Input: part model. Units: mm. Frame: model coordinates. A direction names the side the tool comes from. Coordinates: 2 decimals unless noted, no trailing zeros. Write each loop counter-clockwise with the first axis right and the second up, starting at its lowest first coordinate (ties: lowest second). Pieces come first, ordered by that corner, then holes. Notation, with made-up numbers: (59.5, 54) -> (83.5, 54) arc R17 ccw to (83.5, 80) -> close; hole circle Ø6 at (49.5, 33). An arc over 180 degrees is marked (long way). One line per question, with ' | ' between items. Start each with the question number.
Autodesk Inventor part; units mm, degrees
ref_plane "Arbeitsebene1" through (35.8206, 9.157, 7) normal (0, 0, -1) x (0, 1, 0)
ref_plane "Arbeitsebene2" through (35.8206, 9.157, -7) normal (0, 0, 1) x (1, 0, 0)
ref_plane "YZ Plane" through (0, 0, 0) normal (1, 0, 0) x (0, 1, 0)
sketch "Skizze1" plane through (0, 0, 0) normal (0, 0, 1) x (1, 0, 0)
  circle A0 centre (13.3363, -13.3273) radius 2.25
  circle A1 centre (69.9048, -13.3273) radius 2.25
  line L0 (49.1839, 14.957) -> (45.4022, 8.407)
  line L1 (45.4022, 8.407) -> (37.8389, 8.407)
  line L2 (37.8389, 8.407) -> (34.0573, 14.957)
  circle A2 centre (-86.3794, -2.543) radius 2.1
  line L3 (-65.3794, -2.3212) -> (-80.3794, -2.3212)
  line L4 (-80.3794, -2.3212) -> (-80.3794, 8.457)
  line L5 (-80.3794, 8.457) -> (-86.3794, 8.457)
  line L6 (-86.3794, 8.457) -> (-86.3794, 3.857)
  line L7 (-86.3794, 3.857) -> (-93.3794, 3.857)
  line L8 (-93.3794, 3.857) -> (-93.3794, 8.457)
  line L9 (-93.3794, 8.457) -> (-98.3794, 8.457)
  line L10 (-98.3794, 8.457) -> (-98.3794, -15.043)
  line L11 (-38.3794, -15.043) -> (-98.3794, -15.043)
  spline S0 degree 3 poles (16.2456, -28.9938) (-0.41, -19.3777) (-19.1473, -15.043) (-38.3794, -15.043) knots 1 1 1 1 2 2 2 2
  arc A3 (16.2456, -28.9938) -> (92.3706, 14.957) centre (41.6206, 14.957) ccw
  line L12 (-93.3794, 21.457) -> (-98.3794, 21.457)
  line L13 (-93.3794, 21.457) -> (-93.3794, 26.057)
  line L14 (-93.3794, 26.057) -> (-86.3794, 26.057)
  line L15 (-86.3794, 26.057) -> (-86.3794, 21.457)
  line L16 (-86.3794, 21.457) -> (-80.3794, 21.457)
  line L17 (-80.3794, 32.2352) -> (-80.3794, 21.457)
  line L18 (-65.3794, -4.043) -> (-65.3794, -2.3212)
  line L19 (26.6206, 28.1857) -> (26.6206, 1.7282)
  line L20 (26.6206, 1.7282) -> (16.7234, -4.043)
  line L21 (16.7234, -4.043) -> (-65.3794, -4.043)
  circle A4 centre (41.6206, 14.957) radius 4.1 construction
  line L22 (46.3548, 14.957) -> (43.9877, 19.057)
  line L23 (43.9877, 19.057) -> (39.2534, 19.057)
  line L24 (39.2534, 19.057) -> (36.8863, 14.957)
  line L25 (36.8863, 14.957) -> (39.2534, 10.857)
  line L26 (39.2534, 10.857) -> (43.9877, 10.857)
  line L27 (43.9877, 10.857) -> (46.3548, 14.957)
  arc A5 (92.3706, 14.957) -> (16.2456, 58.9078) centre (41.6206, 14.957) ccw
  spline S1 degree 3 poles (16.2456, 58.9078) (-0.41, 49.2917) (-19.1473, 44.957) (-38.3794, 44.957) knots 1 1 1 1 2 2 2 2
  line L28 (-38.3794, 44.957) -> (-98.3794, 44.957)
  line L29 (-98.3794, 21.457) -> (-98.3794, 44.957)
  line L30 (-65.3794, 32.2352) -> (-80.3794, 32.2352)
  line L31 (-65.3794, 33.957) -> (-65.3794, 32.2352)
  line L32 (16.7234, 33.957) -> (-65.3794, 33.957)
  line L33 (26.6206, 28.1857) -> (16.7234, 33.957)
  circle A6 centre (13.3363, 43.2412) radius 2.25
  circle A7 centre (69.9048, 43.2412) radius 2.25
  circle A8 centre (-86.3794, 32.457) radius 2.1
  line L34 (37.8389, 21.507) -> (34.0573, 14.957)
  line L35 (45.4022, 21.507) -> (37.8389, 21.507)
  line L36 (49.1839, 14.957) -> (45.4022, 21.507)
  point P0 (0, 0)
  dimension "d0" = 8.2
ref_plane "Arbeitsebene1" through (35.8206, 9.157, 7) normal (0, 0, -1) x (0, 1, 0)
ref_plane "Arbeitsebene2" through (35.8206, 9.157, -7) normal (0, 0, 1) x (1, 0, 0)
extrude "Extrusion1" add sketch "Skizze1" against normal up to surface (14 mm away) from surface at 7 contours L0 L1 L2 L34 L35 L36
properties part number "Nutspacker" material "ABS-Kunststoff - Schwarz"
1) First-contact query: P1, Ø3, axis at x = 41, y = 16, coming from the +Z side; P2, Ø2, axis at y = 19.5, z = -4, coming from the -X side. Flat tips, straight axial feed; report the tip coordinate or a pass-through.
2) Access query for faces 1 (the face through (42, 8.407, 0)), 2 (the face through (38.05, 12.94, 0.1)). Directions: +Z, -Z, +X, -X, +Y, -Y. A direction counts if a zero-diameter tool reaches every point of the face in a straight line with its end or side. Return the directions, or none.
3) Section D-D, the plane x = 36. Return loops of the section in (y, z).
4) Section A-A, the plane z = 4.75. Return loops of the section in (x, y).
5) Pull-direction query (X, two-part tool) for faces 3 (the face through (42, 10.857, 0)), 4 (the face through (42, 21.507, 0)), 5 (the face through (47.32, 11.73, 0.1)); classes: released by +X, released by -X, zero draft, split by the parting line, or undercut.
6) Section B-B, the plane x = 42. Return loops of the section in (y, z).
7) Ray query, line 1 (Y direction, x = 40, z = 2.75); line 2 (X direction, y = 12.5, z = -4.5); line 3 (X direction, y = 16.25, z = 3.75). Return the intervals inside material, ascending.
8) Section C-C, the plane y = 12.25. Return loops of the section in (x, z), then the cut area to 3 significant figures.
Answer block:
1) P1: passes through | P2: stops at x = 36.1
2) face 1: +Z, -Z, +X, -X, -Y | face 2: +Z, -Z
3) outline: (11.59, -7) -> (18.32, -7) -> (18.32, 7) -> (11.59, 7) -> close
4) outline: (34.06, 14.96) -> (37.84, 8.41) -> (45.4, 8.41) -> (49.18, 14.96) -> (45.4, 21.51) -> (37.84, 21.51) -> close; hole (36.89, 14.96) -> (39.25, 10.86) -> (43.99, 10.86) -> (46.35, 14.96) -> (43.99, 19.06) -> (39.25, 19.06) -> close
5) face 3: undercut | face 4: zero draft | face 5: released by +X
6) outline: (8.41, -7) -> (10.86, -7) -> (10.86, 7) -> (8.41, 7) -> close; (19.06, -7) -> (21.51, -7) -> (21.51, 7) -> (19.06, 7) -> close
7) line 1: y = 8.41 to 10.86, 19.06 to 21.51 | line 2: x = 35.48 to 38.3, 44.94 to 47.77 | line 3: x = 34.8 to 37.63, 45.61 to 48.44
8) outline: (35.62, -7) -> (38.45, -7) -> (38.45, 7) -> (35.62, 7) -> close; (44.79, -7) -> (47.62, -7) -> (47.62, 7) -> (44.79, 7) -> close | area: 79.2 mm2
